```python
from build123d import *

# Parameters (mm, degrees)
SKETCH1_R           = 8
BOSS_EXTRUDE1_DEPTH = 25
SKETCH2_R           = 4.05
CUT_EXTRUDE1_DEPTH  = 76


with BuildPart() as part:
    # Sketch1 → Boss-Extrude1 (new body)
    with BuildSketch(Plane(origin=(0, 0, 0), x_dir=(1, 0, 0), z_dir=(0, 1, 0))):
        with BuildLine():
            Line((0, 0), (0, 24))
            Line((0, 24), (44, 24))
            Line((44, 24), (44, 33.5))
            ThreePointArc((44, 33.5), (36, 41.5), (44, 49.5))
            Line((44, 49.5), (44, 54))
            Line((44, 54), (44, 66))
            Line((44, 66), (-22, 66))
            Line((-22, 66), (-22, 54))
            Line((-22, 54), (32, 54))
            Line((32, 54), (32, 29))
            Line((32, 29), (-22, 29))
            Line((-22, 29), (-22, -12))
            Line((-22, -12), (44, -12))
            Line((44, -12), (44, 0))
            Line((44, 0), (0, 0))
        make_face()
        with Locations(Location((-11, 12, 0), (0, 0, 270))):
            Circle(SKETCH1_R, mode=Mode.SUBTRACT)
    extrude(amount=BOSS_EXTRUDE1_DEPTH)

    # Sketch2 → Cut-Extrude1 (cut)
    with BuildSketch(Plane(origin=(44, 0, 0), x_dir=(0, 0, -1), z_dir=(1, 0, 0))):
        with Locations((-6, 12.5)):
            Circle(SKETCH2_R)
        with Locations((60, 12.5)):
            Circle(SKETCH2_R)
    extrude(amount=-CUT_EXTRUDE1_DEPTH, mode=Mode.SUBTRACT)


solid = part.part
```
Can you work these out from the model? Positions are in its coordinate system, mm. A direction names the side the tool comes from. Coordinates: 2 decimals unless noted, no trailing zeros. Order: outer loops, then holes, each group sorted by start corner. A loop starts at its lowest first (then second) coordinate and runs counter-clockwise, first axis right, second up. Notation, with made-up numbers: (65.5, 40.25) - (87.5, 40.25) arc R19 cw to (87.5, 62.25) - close; hole circle Ø6 at (70.5, 65.5). An arc over 180 degrees is marked (long way). Answer in a Markdown table with one row per item.
1. Suppose I cut it at C-C (y = 5). Please give me the cut outline in (x, z), and give its area (3 significant figures).
Reply:
| item | result |
|---|---|
| outline | (-22, -66) - (44, -66) - (44, -49.5) arc R8 cw to (44, -33.5) - (44, -24) - (0, -24) - (0, 0) - (44, 0) - (44, 12) - (-22, 12) - (-22, -29) - (32, -29) - (32, -54) - (-22, -54) - close; hole circle Ø16 at (-11, -12) |
| area | 2,440 mm^2 |
2. Suppose I cut it at B-B (z = -60). Please give me the cut outline in (x, y), and give its area (3 significant figures).
Reply:
| item | result |
|---|---|
| outline | (-22, 0) - (44, 0) - (44, 8.45) - (-22, 8.45) - close; (-22, 16.55) - (44, 16.55) - (44, 25) - (-22, 25) - close |
| area | 1,120 mm^2 |
3. If we mould it in two halves opening along Z, with no side actions, what happens to faces 1 (the flat face through (11, 25, -28)), 2 (the flat face through (11, 12, -66)), 3 (the flat face through (22, 12, 0)), 4 (the cylindrical face through (-18.81, 12.32, -13.73))? For each: pulls with the +Z half, pulls with the -Z half, needs draft (parallel to the pull), parting line crosses it, or undercut.
Reply:
| item | result |
|---|---|
| face 1 | needs draft |
| face 2 | pulls with the -Z half |
| face 3 | undercut |
| face 4 | undercut |
4. Suppose I cut it at D-D (x = 22). Please give me the cut outline in (y, z), and give its area (3 significant figures).
Reply:
| item | result |
|---|---|
| outline | (0, -66) - (25, -66) - (25, -54) - (0, -54) - close; (0, -29) - (25, -29) - (25, -24) - (0, -24) - close; (0, 0) - (25, 0) - (25, 12) - (0, 12) - close; hole circle Ø8.1 at (12.5, -60); hole circle Ø8.1 at (12.5, 6) |
| area | 622 mm^2 |
5. If I drill on line 1 along Z through (x, y) = (16, 4.75); line 2 along Z through (x, y) = (-0.5, 19.25); line 3 along Z through (x, y) = (-4, 3), over which ranges is the centre line in solid material (lowest first)?
Reply:
| item | result |
|---|---|
| line 1 | z = -66 to -54, -29 to -24, 0 to 12 |
| line 2 | z = -66 to -54, -29 to 12 |
| line 3 | z = -66 to -54, -29 to -15.87, -8.13 to 12 |
6. Suppose I cut it at A-A (x = -11). Please give me the cut outline in (y, z), and give its area (3 significant figures).
Reply:
| item | result |
|---|---|
| outline | (0, -66) - (25, -66) - (25, -54) - (0, -54) - close; (0, -29) - (25, -29) - (25, -20) - (0, -20) - close; (0, -4) - (25, -4) - (25, 12) - (0, 12) - close; hole circle Ø8.1 at (12.5, -60); hole circle Ø8.1 at (12.5, 6) |
| area | 822 mm^2 |
7. For faces 5 (the flat face through (5, 12, -54)), 6 (the flat face through (44, 10, 10)), 7 (the flat face through (0, 12, -12)), which set-ups out of +Z, -Z, +X, -X, +Y, -Y let a thin tool reach every point of the face, with its end or its side?
Reply:
| item | result |
|---|---|
| face 5 | -X, +Y, -Y |
| face 6 | +Z, -Z, +X, +Y, -Y |
| face 7 | +X, +Y, -Y |
8. For pin 1 (18.5 mm diameter, centred on x = -11, z = -12, fed in from +Y); pin 2 (6 mm diameter, centred on y = 13.5, z = -5.5, fed in from +X), each with a flat end and sliding along its axis, tell me the tip position at first contact or that it passes through.
Reply:
| item | result |
|---|---|
| pin 1 | stops at y = 25 |
| pin 2 | stops at x = 0 |
